from build123d import *

# Parameters (mm, degrees)
F4_DEPTH = 6.35
F5_DEPTH = 3.175
F6_DEPTH = 6.35
F7_DEPTH = 6.35


with BuildPart() as f4:
    # F0 (on Top) → F4 (new body)
    with BuildSketch(Plane.XY):
        with BuildLine():
            Line((0, 65.86501), (-12.691889, 44.004165))
            add(Edge.make_bspline(
                [(-12.691889, 44.004165), (0, 41.807882), (8.420921, 39.781306), (19.231755, 33.027414)],
                knots=[0, 0, 0, 0, 33.758082, 33.758082, 33.758082, 33.758082], degree=3))
            add(Edge.make_bspline(
                [(9.615878, 49.446212), (13.190391, 43.027269), (16.764905, 36.608325), (19.231755, 33.027414)],
                knots=[19.027402, 19.027402, 19.027402, 19.027402, 38.054804, 38.054804, 38.054804, 38.054804], degree=3))
            Line((9.615878, 49.446212), (0, 65.86501))
        make_face()
        with BuildLine():
            add(Edge.make_bspline(
                [(0, 65.86501), (2.46685, 62.284099), (6.041364, 55.865156), (9.615878, 49.446212)],
                knots=[0, 0, 0, 0, 19.027402, 19.027402, 19.027402, 19.027402], degree=3))
            Line((0, 65.86501), (9.615878, 49.446212))
        make_face()
        with BuildLine():
            add(Edge.make_bspline(
                [(9.615878, 49.446212), (13.190391, 43.027269), (16.764905, 36.608325), (19.231755, 33.027414)],
                knots=[19.027402, 19.027402, 19.027402, 19.027402, 38.054804, 38.054804, 38.054804, 38.054804], degree=3))
            Line((19.231755, 33.027414), (9.615878, 49.446212))
        make_face()
    extrude(amount=F4_DEPTH)

    # F3 (on Top) → F5 (join)
    with BuildSketch(Plane.XY):
        Polygon((43.985669, -3.733072), (0, 73.194362), (-44.357441, -3.733072), align=None)
    extrude(amount=F5_DEPTH)

    # F2 (on Top) → F6 (join)
    with BuildSketch(Plane.XY):
        with BuildLine():
            Line((38.493596, 0), (24.638867, 22.391399))
            add(Edge.make_bspline(
                [(24.638867, 22.391399), (26.498249, 15.807372), (12.989721, 2.810146), (-8.79713, 0)],
                knots=[0, 0, 0, 0, 40.241032, 40.241032, 40.241032, 40.241032], degree=3))
            Line((-8.79713, 0), (38.493596, 0))
        make_face()
    extrude(amount=F6_DEPTH)

    # F1 (on Top) → F7 (join)
    with BuildSketch(Plane.XY):
        with BuildLine():
            Line((-15.045927, 39.76772), (-37.978165, 0))
            add(Edge.make_bspline(
                [(-37.978165, 0), (-24.740312, -0.17884), (-3.689409, 7.116403), (0, 15.49142)],
                knots=[0, 0, 0, 0, 41.016157, 41.016157, 41.016157, 41.016157], degree=3))
            add(Edge.make_bspline(
                [(-15.045927, 39.76772), (0, 30.680645), (2.194603, 18.867477), (0, 15.49142)],
                knots=[0, 0, 0, 0, 28.560788, 28.560788, 28.560788, 28.560788], degree=3))
        make_face()
    extrude(amount=F7_DEPTH)


solid = f4.part
The model under review builds one solid part; all positions refer to its coordinate system, in mm. A direction names the side the tool comes from. Round coordinates to 2 decimals unless told otherwise and drop trailing zeros. Loops run counter-clockwise (first coordinate to the right, second up) from the corner with the lowest first, then second, coordinate; pieces in that order, holes last. Notation, with made-up numbers: M 6.25,62 L 44.25,62 A23 ccw 44.25,91 Z; hole C 46,7 d1. An arc over 180 degrees is marked long. Answer as CSV lines item,"result". Start each with the question number.
Item 1: Consider section A-A (z = 5). State how many separate pieces and enclosed holes the cut face has, then the cut area to 3 significant figures.
Item 2: For faces 5 (the face through (31.663, 11.039, 4.74)), 6 (the face through (15, 0, 5)), 7 (the face through (-26.352, 20.162, 4.74)), 8 (the face through (-1, 27, 0)), 9 (the face through (3, 50, 6.35)), list the 3-axis set-ups (+Z, -Z, +X, -X, +Y, -Y) from which the entire face can be reached by the end or side of a thin tool; tool diameter is ignored.
Item 3: Consider section B-B (y = 48). Write out the cut boundary in (x, z) (3 decimals), then the cut area to 3 significant figures.
Item 4: Consider section D-D (y = 68). Write out the cut boundary in (x, z) (3 decimals), then the cut area to 3 significant figures.
Item 5: Insertion check: P1, Ø3, axis at y = 23.5, z = 5.5, coming from the +X side; P2, Ø1.6, axis at x = 22, z = 5, coming from the -Y side; P3, Ø1, axis at x = 3, y = 27.5, coming from the +Z side (3 decimals). Each pin has a flat end and moves straight along its axis. Give the tip position at first contact, or say it passes through.
Item 6: Consider section C-C (x = 36). Write out the cut boundary in (y, z) (3 decimals), then the cut area to 3 significant figures.
Item 7: Wall thickness on line 1 (Z direction, x = 13.5, y = 28.5) (3 decimals); line 2 (X direction, y = 14, z = 4.75) (3 decimals); line 3 (Y direction, x = 11, z = 4.5): over which ranges is each line inside the solid? List them lowest first. Write a range as [from, to].
Item 8: Mouldability with a two-part tool opening along X and no side actions: class faces 1 (the face through (3, 21, 3.175)), 2 (the face through (22.3, 34.19, 1.57)), 3 (the face through (-6.257, 55.088, 4.74)), 4 (the face through (-1, -3.733, 2)) as released by +X, released by -X, zero draft, split by the parting line, or undercut.
Answer:
1,separate pieces,"3"
1,enclosed holes,"0"
1,area,"1,530 mm^2"
2,face 5,"+Z, +X, +Y"
2,face 6,"+Z, +X, -X, -Y"
2,face 7,"+Z, -X, +Y"
2,face 8,"-Z, +X, -X, +Y, -Y"
2,face 9,"+Z, +X, -X, +Y, -Y"
3,outline,"M -14.527,0 L 14.406,0 L 14.406,3.175 L 10.463,3.175 L 10.463,6.35 L -10.372,6.35 L -10.372,3.175 L -14.527,3.175 Z"
3,area,"158 mm^2"
4,outline,"M -2.995,0 L 2.97,0 L 2.97,3.175 L -2.995,3.175 Z"
4,area,"18.9 mm^2"
5,P1,"stops at x = 24.88"
5,P2,"stops at y = 0"
5,P3,"stops at z = 3.175"
6,outline,"M -3.733,0 L 10.233,0 L 10.233,3.175 L 4.03,3.175 L 4.03,6.35 L 0,6.35 L 0,3.175 L -3.733,3.175 Z"
6,area,"57.1 mm^2"
7,line 1,"z = [0, 3.175]"
7,line 2,"x = [-29.905, -0.844], [21.394, 29.831]"
7,line 3,"y = [0, 6.12], [37.5, 47.08]"
8,face 1,"undercut"
8,face 2,"released by +X"
8,face 3,"released by -X"
8,face 4,"zero draft"
